Part print with two shaded views. Sizes in mm from the minimum x, y, z corner. Round coordinates to 2 decimals unless told otherwise and drop trailing zeros. Loops run counter-clockwise (first coordinate to the right, second up) from the corner with the lowest first, then second, coordinate; pieces in that order, holes last. Notation, with made-up numbers: (-33.75, -35) - (-0.75, -35) arc R25 ccw to (-0.75, -9) - close; hole circle Ø8 at (-23.75, 56.25). An arc over 180 degrees is marked (long way). Put each result on its own line as item: value. Start each with the question number.
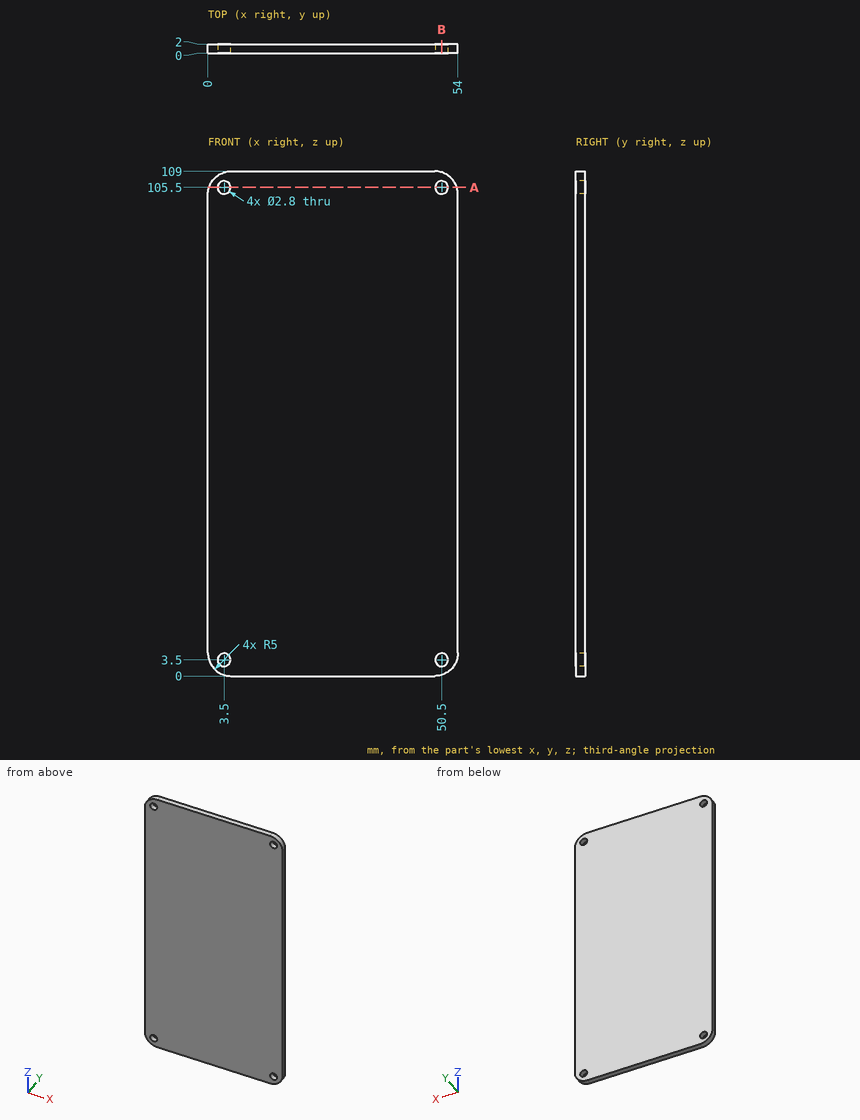
1) Slice it at A-A, the plane z = 105.5. Write the cut outline in (x, y).
2) Drop a flat-ended pin along its axis: pin 1 Ø5 at (x, z) = (16, 34) entering from -Y. Give the stop position or say it passes through.
3) Drill centre lines: line 1 (Z direction, x = 3.5, y = 1.25); line 2 (Z direction, x = 51, y = 1.3); line 3 (X direction, y = 0.6, z = 105.5). Where is each one in solid material? Low to high. Write a range as [from, to].
4) Slice it at B-B, the plane x = 50.5. Write the cut outline in (y, z), and give its area (3 significant figures).
Taken from the geometry:
1. outline: (0.23, 0) - (2.1, 0) - (2.1, 2) - (0.23, 2) - close; (4.9, 0) - (49.1, 0) - (49.1, 2) - (4.9, 2) - close; (51.9, 0) - (53.77, 0) - (53.77, 2) - (51.9, 2) - close
2. pin 1: stops at y = 0
3. line 1: z = [0.23, 2.1], [4.9, 104.1], [106.9, 108.77]
3. line 2: z = [0.42, 2.19], [4.81, 104.19], [106.81, 108.58]
3. line 3: x = [0.23, 2.1], [4.9, 49.1], [51.9, 53.77]
4. outline: (0, 0.23) - (2, 0.23) - (2, 2.1) - (0, 2.1) - close; (0, 4.9) - (2, 4.9) - (2, 104.1) - (0, 104.1) - close; (0, 106.9) - (2, 106.9) - (2, 108.77) - (0, 108.77) - close
4. area: 206 mm2
